Answer from the drawing. Dimensions are ordinates in mm from the lowest x, y and z of the part. A direction names the side the tool comes from. Round coordinates to 2 decimals unless told otherwise and drop trailing zeros. Order: outer loops, then holes, each group sorted by start corner. A loop starts at its lowest first (then second) coordinate and runs counter-clockwise, first axis right, second up.
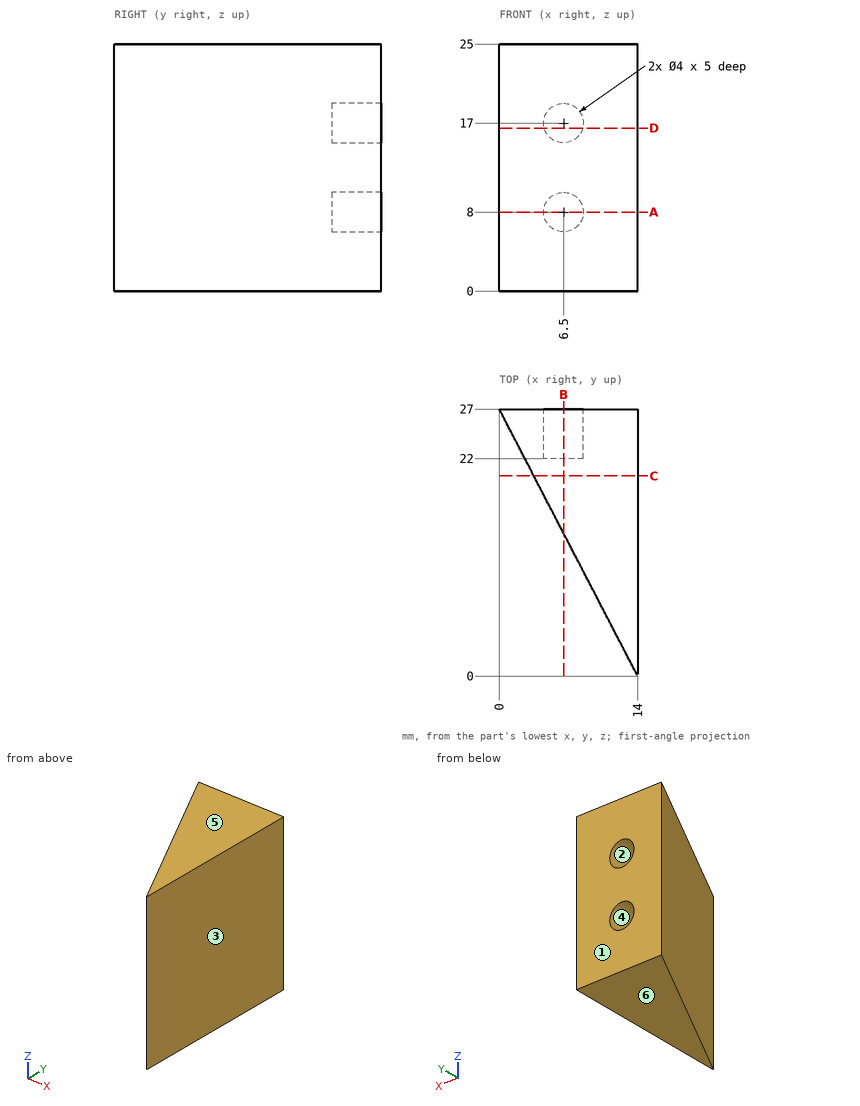
Q1. A cutting plane is placed at A-A, the plane z = 8. Give the vertices of the cut face in (x, y), plus the area to 3 significant figures.
Outcome:
outline: (0, 27) - (14, 0) - (14, 27) - (8.5, 27) - (8.5, 22) - (4.5, 22) - (4.5, 27) - close
area: 169 mm2
Q2. A cutting plane is placed at B-B, the plane x = 6.5. Give the vertices of the cut face in (y, z), plus the area to 3 significant figures.
Outcome:
outline: (14.46, 0) - (27, 0) - (27, 6) - (22, 6) - (22, 10) - (27, 10) - (27, 15) - (22, 15) - (22, 19) - (27, 19) - (27, 25) - (14.46, 25) - close
area: 273 mm2
Q3. A cutting plane is placed at D-D, the plane z = 16.5. Give the vertices of the cut face in (x, y), plus the area to 3 significant figures.
Outcome:
outline: (0, 27) - (14, 0) - (14, 27) - (8.44, 27) - (8.44, 22) - (4.56, 22) - (4.56, 27) - close
area: 170 mm2
Q4. For a pull along Z with two mould halves and no side action, classify the marked faces 3, 4, 5 and 6 as released by +Z, released by -Z, zero draft, split by the parting line, or undercut.
Outcome:
face 3: zero draft
face 4: undercut
face 5: released by +Z
face 6: released by -Z
Q5. For the marked faces 1 and 2, determine the directions among +Z, -Z, +X, -X, +Y, -Y from which every point of the face is accessible in a straight line to the end or side of a thin tool.
Outcome:
face 1: +Z, -Z, +X, -X, +Y
face 2: +Y
Q6. A cutting plane is placed at C-C, the plane y = 20.25. Give the vertices of the cut face in (x, z).
Outcome:
outline: (3.5, 0) - (14, 0) - (14, 25) - (3.5, 25) - close
Q7. Flat-ended cylindrical pins translate along their axes: pin 1 (3 mm diameter, centred on y = 5, z = 12.5, fed in from -X); pin 2 (1 mm diameter, centred on x = 8.5, y = 7.5, fed in from +Z); pin 3 (5 mm diameter, centred on y = 11.5, z = 16, fed in from -X); pin 4 (3.5 mm diameter, centred on x = 6.5, z = 17, fed in from -Y). Find the tip coordinate at first contact, or state that the pin passes through.
Outcome:
pin 1: stops at x = 10.63
pin 2: passes through
pin 3: stops at x = 6.74
pin 4: stops at y = 11.09
Q8. Straight lines are drawn through the part: probe 1 along X at (y, z) = (24.9, 17); probe 2 along X at (y, z) = (24.4, 17); probe 3 along Y at (x, z) = (9, 1.5). For each, find the intervals that lie inside material, in ascending order.
Outcome:
probe 1: x = 1.09 to 4.5, 8.5 to 14
probe 2: x = 1.35 to 4.5, 8.5 to 14
probe 3: y = 9.64 to 27
